```python
from build123d import *

# Parameters (mm, degrees)
SKETCH1_R                           = 2.159
BOSS_EXTRUDE1_DEPTH                 = 1.575
SKETCH2_W                           = 93.457658642
SKETCH2_H                           = 6.602
CUT_EXTRUDE1_DEPTH                  = 65.362755899
CUT_EXTRUDE2_DEPTH                  = 60.755092082
CUT_EXTRUDE3_DEPTH                  = 60.755092082
SKETCH6_R                           = 0.8382
CUT_EXTRUDE4_DEPTH                  = 2.54
SKETCH7_W                           = 65.648
SKETCH7_H                           = 12
CUT_EXTRUDE5_DEPTH                  = 59.286069146
SKETCH11_R                          = 0.270027719
ID_HOLE_DEPTH                       = 59.286069146
SKETCH12_W                          = 2.575
SKETCH12_H                          = 5
NOTCH_FOR_BPR_TOP_VIEW_DEPTH        = 59.286069146
SKETCH14_W                          = 2.575
SKETCH14_H                          = 12.502619879
NOTCH_FOR_BPL_TOP_VIEW_DEPTH        = 59.286069146
SKETCH17_W                          = 73.57
SKETCH17_H                          = 1
CREATE_LIP_FOR_M3_SPACER_HOLE_DEPTH = 1.575
SKETCH15_R                          = 1.6
HOLE_FOR_M3_SPACER_DEPTH            = 59.977069112
SKETCH19_W                          = 6.013982762
SKETCH19_H                          = 1.7
SKETCH19_W_2                        = 9.814467677
CUT_EXTRUDE7_DEPTH                  = 59.977069112


with BuildPart() as part:
    # Sketch1 → Boss-Extrude1 (new body)
    with BuildSketch(Plane(origin=(0, 0, 0), x_dir=(1, 0, 0), z_dir=(0, 1, 0))):
        Polygon((44.351293299, -40.014412246), (37.136293299, -40.014412246), (37.136293299, -46.615946892), (29.968293307, -46.615946892), (-30.083706693, -46.615946892), (-36.433706701, -46.615946892), (-36.433706701, -40.014412246), (-43.648706701, -40.014412246), (-43.648706701, -30.885946892), (-43.648706701, -29.647946892), (-42.378706693, -29.615946892), (-32.472706701, -29.647946892), (-32.472706701, -10.370428445), (-12.155556701, -10.370428445), (-12.155556701, -34.615947016), (-11.557706701, -34.615947016), (12.260293299, -34.615947016), (12.858143299, -34.615947016), (12.858143299, -10.370428445), (33.175293299, -10.370428445), (33.175293299, -12.929386892), (33.175293299, -29.647946892), (38.746293307, -29.615946892), (42.351293307, -29.615946892), (44.351293299, -29.615946892), (44.351293299, -31.651946892), align=None)
        with Locations(Location((-19.648556701, -28.76738335, 0), (0, 0, 270))):
            Circle(SKETCH1_R, mode=Mode.SUBTRACT)
        with Locations(Location((-19.648556701, -20.63938335, 0), (0, 0, 270))):
            Circle(SKETCH1_R, mode=Mode.SUBTRACT)
        with Locations(Location((20.351397299, -20.63938335, 0), (0, 0, 270))):
            Circle(SKETCH1_R, mode=Mode.SUBTRACT)
        with Locations(Location((20.351397299, -28.76738335, 0), (0, 0, 270))):
            Circle(SKETCH1_R, mode=Mode.SUBTRACT)
    extrude(amount=BOSS_EXTRUDE1_DEPTH)

    # Sketch2 → Cut-Extrude1 (cut, through all)
    with BuildSketch(Plane.XZ):
        with Locations((-2.377536022, 43.315412246)):
            Rectangle(SKETCH2_W, SKETCH2_H)
    extrude(amount=-CUT_EXTRUDE1_DEPTH, mode=Mode.SUBTRACT)

    # Sketch3 → Cut-Extrude2 (cut, through all)
    with BuildSketch(Plane.XZ):
        Polygon((-41.504650493, 40.014412246), (-41.504650493, 29.618770413), (-34.629650483, 29.640979175), (-34.629650483, 8.976090323), (-48.128778183, 8.976090323), (-48.128778183, 40.014412246), align=None)
    extrude(amount=-CUT_EXTRUDE2_DEPTH, mode=Mode.SUBTRACT)

    # Sketch4 → Cut-Extrude3 (cut, through all)
    with BuildSketch(Plane.XZ):
        Polygon((42.351293299, 40.014412246), (42.351293299, 32.420104455), (42.351293299, 29.615946892), (35.476293307, 29.615946892), (35.476293307, 10.370428445), (54.710892309, 10.370428445), (54.710892309, 40.014412246), align=None)
    extrude(amount=-CUT_EXTRUDE3_DEPTH, mode=Mode.SUBTRACT)

    # Sketch6 → Cut-Extrude4 (cut)
    with BuildSketch(Plane(origin=(0, 0, 0), x_dir=(-1, 0, 0), z_dir=(0, -1, 0))):
        with Locations(Location((27.141556701, -35.947946892, 0), (0, 0, 90))):
            Circle(SKETCH6_R)
        with Locations(Location((27.141556701, -25.025946892, 0), (0, 0, 90))):
            Circle(SKETCH6_R)
        with Locations(Location((14.695556701, -25.025946892, 0), (0, 0, 90))):
            Circle(SKETCH6_R)
        with Locations(Location((-15.398143299, -25.025946892, 0), (0, 0, 90))):
            Circle(SKETCH6_R)
        with Locations(Location((-27.844397299, -25.025946892, 0), (0, 0, 90))):
            Circle(SKETCH6_R)
        with Locations(Location((-27.844397299, -35.947946892, 0), (0, 0, 90))):
            Circle(SKETCH6_R)
    extrude(amount=-CUT_EXTRUDE4_DEPTH, mode=Mode.SUBTRACT)

    # Sketch7 → Cut-Extrude5 (cut, through all)
    with BuildSketch(Plane.XZ):
        with Locations((0.351293299, 16.370428445)):
            Rectangle(SKETCH7_W, SKETCH7_H)
    extrude(amount=-CUT_EXTRUDE5_DEPTH, mode=Mode.SUBTRACT)

    # Sketch11 → ID HOLE (cut, through all)
    with BuildSketch(Plane(origin=(0, 1.575, 0), x_dir=(1, 0, 0), z_dir=(0, 1, 0))):
        with Locations(Location((-40.144429695, -32.22382703, 0), (0, 0, 270))):
            Circle(SKETCH11_R)
    extrude(amount=-ID_HOLE_DEPTH, mode=Mode.SUBTRACT)

    # Sketch12 → Notch for BPR (TOP VIEW) (cut, through all)
    with BuildSketch(Plane(origin=(0, 0, 0), x_dir=(-1, 0, 0), z_dir=(0, -1, 0))):
        with Locations((35.201150493, -32.134973926)):
            Rectangle(SKETCH12_W, SKETCH12_H)
    extrude(amount=-NOTCH_FOR_BPR_TOP_VIEW_DEPTH, mode=Mode.SUBTRACT)

    # Sketch14 → Notch for BPL (TOP VIEW) (cut, through all)
    with BuildSketch(Plane(origin=(0, 0, 0), x_dir=(-1, 0, 0), z_dir=(0, -1, 0))):
        with Locations((-36.253849507, -28.621738385)):
            Rectangle(SKETCH14_W, SKETCH14_H)
    extrude(amount=-NOTCH_FOR_BPL_TOP_VIEW_DEPTH, mode=Mode.SUBTRACT)

    # Sketch17 → Create Lip for M3 Spacer Hole (add)
    with BuildSketch(Plane.XZ):
        with Locations((0.351293299, 40.514412246)):
            Rectangle(SKETCH17_W, SKETCH17_H)
    extrude(amount=-CREATE_LIP_FOR_M3_SPACER_HOLE_DEPTH)

    # Sketch15 → HOLE for M3 Spacer (cut, through all)
    with BuildSketch(Plane.XZ):
        with Locations(Location((-0.006565304, 37.835831124, 0), (0, 0, 270))):
            Circle(SKETCH15_R)
        with Locations(Location((-33.429715371, 37.835831124, 0), (0, 0, 270))):
            Circle(SKETCH15_R)
        with Locations(Location((34.851293299, 37.835831124, 0), (0, 0, 270))):
            Circle(SKETCH15_R)
    extrude(amount=-HOLE_FOR_M3_SPACER_DEPTH, mode=Mode.SUBTRACT)

    # Sketch19 → Cut-Extrude7 (cut, through all)
    with BuildSketch(Plane.XZ):
        with Locations((40.047258401, 28.864412246)):
            Rectangle(SKETCH19_W, SKETCH19_H)
        with Locations((-40.560325306, 28.864412246)):
            Rectangle(SKETCH19_W_2, SKETCH19_H)
    extrude(amount=-CUT_EXTRUDE7_DEPTH, mode=Mode.SUBTRACT)


solid = part.part
```
Verification items for the finished model (mm, model axes). A direction names the side the tool comes from. Give positions to 0.01 mm unless a question says otherwise; leave off trailing zeros. Loops run counter-clockwise (first coordinate to the right, second up) from the corner with the lowest first, then second, coordinate; pieces in that order, holes last. Notation, with made-up numbers: M 28.5,-27.5 L 34.5,-27.5 A31 cw 34.5,-1.5 Z; hole C 86.25,-3.5 d2. An arc over 180 degrees is marked long. Return JSON: item names as keys, results as strings.
1) Gauge pin test, flat ends, axial feed: P1, Ø0.5, axis at x = 36.5, y = 0.5, coming from the -Z side; P2, Ø0.8, axis at x = -35, y = 0.5, coming from the -Z side (3 decimals); P3, Ø0.5, axis at y = 1, z = 29, coming from the +X side. Record the tip position at first contact, or that the pin passes through.
Findings:
{"P1": "stops at z = 34.87", "P2": "stops at z = 34.635", "P3": "stops at x = 33.18"}
2) Material ranges on L1, parallel to X at y = 0.25, z = 32.75; L2, parallel to Z at x = 35, y = 1.4; L3, parallel to X at y = 1.4, z = 30.75, recorded low to high. Write a range as [from, to].
Findings:
{"L1": "x = [-41.5, -36.49], [-33.91, -12.16], [12.86, 34.97], [37.54, 42.35]", "L2": "z = [34.87, 36.24], [39.43, 41.01]", "L3": "x = [-41.5, -36.49], [-33.91, -20.5], [-18.79, -12.16], [12.86, 19.5], [21.21, 34.97], [37.54, 42.35]"}
3) Section check B-B, the plane x = -3. Enter the section's corners in (y, z) (3 decimals), and give its area (3 significant figures).
Findings:
{"outline": "M 0,34.616 L 1.575,34.616 L 1.575,41.014 L 0,41.014 Z", "area": "10.1 mm2"}
4) Mould release check, pull along X, two halves, no side actions. Record for faces 3 (the flat face through (-39, 1, 40.014)), 4 (the flat face through (-32.473, 1, 26)), 5 (the flat face through (33.175, 1, 26)), 6 (the cylindrical face through (33.29, 0.78, 38.18)): released by +X, released by -X, zero draft, split by the parting line, or undercut.
Findings:
{"face 3": "zero draft", "face 4": "released by -X", "face 5": "released by +X", "face 6": "undercut"}
5) Section check A-A, the plane z = 27.75. Enter the section's corners in (x, y) (3 decimals), and give its area (3 significant figures).
Findings:
{"outline": "M -32.473,0 L -21.553,0 L -21.553,1.575 L -32.473,1.575 Z; M -17.744,0 L -12.156,0 L -12.156,1.575 L -17.744,1.575 Z; M 12.858,0 L 18.447,0 L 18.447,1.575 L 12.858,1.575 Z; M 22.256,0 L 33.175,0 L 33.175,1.575 L 22.256,1.575 Z", "area": "52.0 mm2"}
6) Section check C-C, the plane y = 0.9. Count the separate pieces of the cut face and the enclosed holes in it, and give its area (3 significant figures).
Findings:
{"separate pieces": "1", "enclosed holes": "12", "area": "1,020 mm2"}
7) Tool access check on faces 1 (the flat face through (36, 1, 34.873)), 2 (the cylindrical face through (28.411, 0.776, 25.644)). Record the directions out of +Z, -Z, +X, -X, +Y, -Y that give a thin tool (end or side, any length) a straight path to the whole face; none if there is none.
Findings:
{"face 1": "-Z, +Y, -Y", "face 2": "+Y, -Y"}
